```python
from build123d import *

# Parameters (mm, degrees)
SKETCH1_W           = 11
SKETCH1_H           = 22
BOSS_EXTRUDE1_DEPTH = 5
SKETCH3_W           = 21
SKETCH3_H           = 175
BOSS_EXTRUDE2_DEPTH = 10
CUT_EXTRUDE1_DEPTH  = 151
SKETCH5_R           = 5
CUT_EXTRUDE2_DEPTH  = 15
CUT_EXTRUDE3_START  = -2.25
SKETCH6_W           = 12
SKETCH6_H           = 128.5
SKETCH6_H_2         = 7.5
CUT_EXTRUDE3_DEPTH  = 2.25


with BuildPart() as part:
    # Sketch1 → Boss-Extrude1 (new body)
    with BuildSketch(Plane(origin=(0, 0, 0), x_dir=(0, 1, 0), z_dir=(0, 0, 1))):
        Rectangle(SKETCH1_W, SKETCH1_H)
    extrude(amount=BOSS_EXTRUDE1_DEPTH)


with BuildPart() as body_2:
    # Sketch3 → Boss-Extrude2 (new body)
    with BuildSketch(Plane(origin=(0, 22, 0), x_dir=(-1, 0, 0), z_dir=(0, 1, 0))):
        with Locations((0, 162.5)):
            Rectangle(SKETCH3_W, SKETCH3_H)
    extrude(amount=-BOSS_EXTRUDE2_DEPTH)


    add(part.part)  # loft1 joins it to this body
    # loft from a face of the part (loft1)
    loft([body_2.faces().sort_by_distance((0, 12, 162.5))[0], body_2.faces().sort_by_distance((0, 0, 5))[0]])

    # Sketch4 → Cut-Extrude1 (cut)
    with BuildSketch(Plane.XY.offset(250)):
        Polygon((-3.25, 22), (-3.25, 19.75), (-6, 19.75), (-6, 15.5), (6, 15.5), (6, 19.75), (3.25, 19.75), (3.25, 22), align=None)
    extrude(amount=-CUT_EXTRUDE1_DEPTH, mode=Mode.SUBTRACT)

    # Sketch5 → Cut-Extrude2 (cut)
    with BuildSketch(Plane(origin=(0, 22, 0), x_dir=(-1, 0, 0), z_dir=(0, 1, 0))):
        with Locations(Location((0, 91.5, 0), (0, 0, 90))):
            Circle(SKETCH5_R)
    extrude(amount=-CUT_EXTRUDE2_DEPTH, mode=Mode.SUBTRACT)

    # Sketch6 → Cut-Extrude3 (cut)
    with BuildSketch(Plane(origin=(0, 22, 0), x_dir=(-1, 0, 0), z_dir=(0, 1, 0)).offset(CUT_EXTRUDE3_START)):
        with Locations((0, 178.25)):
            Rectangle(SKETCH6_W, SKETCH6_H)
        with Locations((0, 102.75)):
            Rectangle(SKETCH6_W, SKETCH6_H_2)
    extrude(amount=CUT_EXTRUDE3_DEPTH, mode=Mode.SUBTRACT)


solid = body_2.part
```
Can you work these out from the model? Positions are in its coordinate system, mm. A direction names the side the tool comes from. Coordinates: 2 decimals unless noted, no trailing zeros. Answer as a JSON object with one key per item and string values.
1) Thinking about a two-plate mould opening in X: for faces 4 (the face through (0, 7, 91)), 5 (the face through (-10.5, 17, 161)), 6 (the face through (0, 0, 0)), which applies, pulls with the +X half, pulls with the -X half, needs draft (parallel to the pull), parting line crosses it, or undercut?
Results:
{"face 4": "undercut", "face 5": "pulls with the -X half", "face 6": "needs draft"}
2) For P1, Ø0.8, axis at x = 4, z = 247.5, coming from the -Y side; P2, Ø11, axis at y = 19, z = 142.5, coming from the +X side; P3, Ø8, axis at x = 4.5, y = 18, coming from the -Z side, each with a flat end and sliding along its axis, tell me the tip position at first contact or that it passes through.
Results:
{"P1": "stops at y = 11.79", "P2": "stops at x = 10.5", "P3": "stops at z = 75"}
3) If I drill on line 1 (Z direction, x = 5.5, y = 20); line 2 (X direction, y = 20.25, z = 228); line 3 (X direction, y = 14.5, z = 91.5), over which ranges is the centre line in solid material (lowest first)?
Results:
{"line 1": "z = 75 to 99, 106.5 to 114, 242.5 to 250", "line 2": "x = -10.5 to -6, 6 to 10.5", "line 3": "x = -10.5 to -5, 5 to 10.5"}
4) For faces 1 (the face through (0, 17, 75)), 2 (the face through (6, 19, 176)), 3 (the face through (10.5, 17, 161)), which set-ups out of +Z, -Z, +X, -X, +Y, -Y let a thin tool reach every point of the face, with its end or its side?
Results:
{"face 1": "-Z, +X, -X, +Y", "face 2": "none", "face 3": "+Z, -Z, +X, +Y"}
